Read the model definition and answer for the solid it produces. Units are mm, in the model's axes. Coordinates: 2 decimals unless noted, no trailing zeros.
Q1. The mould has two halves that part along X. Classify faces 1 (the face through (-47.083, -0.014, 44.087)), 2 (the face through (-70.4, 26.4, 2.6)), 3 (the face through (-85.32, 15.44, -56.24)): pulls with the +X half, pulls with the -X half, needs draft (parallel to the pull), parting line crosses it, or undercut.
Q2. Straight lines are drawn through the part: line 1 (Z direction, x = -100, y = 10); line 2 (Z direction, x = -55.5, y = 20.75); line 3 (Z direction, x = -84, y = 9.75). For each, find the intervals that lie inside material, in ascending order.
Q3. Flat-ended cylindrical pins translate along their axes: P1, Ø1.5, axis at x = -83, y = 21, coming from the +Z side; P2, Ø8.5, axis at x = -54.5, z = -26.5, coming from the +Y side; P3, Ø10, axis at x = -59.5, y = 7.5, coming from the +Z side. Find the tip coordinate at first contact, or state that the pin passes through.
Q4. Section A-A (y = 19) is taken. Count the separate pieces of the cut face and the enclosed holes in it, then the cut area to 3 significant figures.
from build123d import *

# Parameters (mm, degrees)
BOSS_EXTRUDE1_DEPTH = 1
BOSS_EXTRUDE2_DEPTH = 25.4
SKETCH4_R           = 14.351
CUT_EXTRUDE1_DEPTH  = 25.4
SKETCH4_4_R         = 19.177
CUT_EXTRUDE2_DEPTH  = 22.225
LPATTERN1_COUNT     = 3
LPATTERN1_PITCH     = 78
SPLIT3_START        = -1
SPLIT3_DEPTH        = 27.4


# Read off the part's stored shape, not the designer's step: Split3
with BuildPart() as part:
    # Sketch1 → Boss-Extrude1 (new, symmetric)
    with BuildSketch(Plane(origin=(0, 0, 0), x_dir=(1, 0, 0), z_dir=(0, 1, 0))):
        Polygon((118, 0), (-118, 0), (-118, -67.135), (118, -75), align=None)
        Polygon((-118, 67.135), (-118, 0), (118, 0), (118, 75), align=None)
    extrude(amount=BOSS_EXTRUDE1_DEPTH, both=True)

    # Sketch3 → Boss-Extrude2 (add)
    with BuildSketch(Plane(origin=(0, 1, 0), x_dir=(1, 0, 0), z_dir=(0, 1, 0))):
        Polygon((-84.001477372, 20.6375), (-73.002954744, 39.6875), (-84.001477372, 58.7375), (-105.998522628, 58.7375), (-116.997045256, 39.6875), (-105.998522628, 20.6375), align=None)
        Polygon((-38.632571531, 19.84375), (-49.631094159, 0.79375), (-71.628139415, 0.79375), (-82.626662043, 19.84375), (-71.628139415, 38.89375), (-49.631094159, 38.89375), align=None)
        Polygon((-84.001477372, -19.05), (-73.002954744, 0), (-84.001477372, 19.05), (-105.998522628, 19.05), (-116.997045256, 0), (-105.998522628, -19.05), align=None)
        Polygon((-105.998522628, -58.7375), (-84.001477372, -58.7375), (-73.002954744, -39.6875), (-84.001477372, -20.6375), (-105.998522628, -20.6375), (-116.997045256, -39.6875), align=None)
        Polygon((-71.628139415, -38.89375), (-49.631094159, -38.89375), (-38.632571531, -19.84375), (-49.631094159, -0.79375), (-71.628139415, -0.79375), (-82.626662043, -19.84375), align=None)
    boss_extrude2 = extrude(amount=BOSS_EXTRUDE2_DEPTH)

    # Sketch4 → Cut-Extrude1 (cut)
    with BuildSketch(Plane(origin=(0, 26.4, 0), x_dir=(1, 0, 0), z_dir=(0, 1, 0))):
        with Locations(Location((-95, 0, 0), (0, 0, 270))):
            Circle(SKETCH4_R)
        with Locations(Location((-95, -39.6875, 0), (0, 0, 270))):
            Circle(SKETCH4_R)
        with Locations(Location((-95, 39.6875, 0), (0, 0, 90))):
            Circle(SKETCH4_R)
        with Locations(Location((-60.629616787, 19.84375, 0), (0, 0, 270))):
            Circle(SKETCH4_R)
        with Locations(Location((-60.629616787, -19.84375, 0), (0, 0, 90))):
            Circle(SKETCH4_R)
    cut_extrude1 = extrude(amount=-CUT_EXTRUDE1_DEPTH, mode=Mode.SUBTRACT)

    # Sketch4<4> → Cut-Extrude2 (cut)
    with BuildSketch(Plane(origin=(0, 26.4, 0), x_dir=(1, 0, 0), z_dir=(0, 1, 0))):
        with Locations((-95, 0)):
            Circle(SKETCH4_4_R)
        with Locations((-95, -39.6875)):
            Circle(SKETCH4_4_R)
        with Locations((-95, 39.6875)):
            Circle(SKETCH4_4_R)
        with Locations((-60.629616787, 19.84375)):
            Circle(SKETCH4_4_R)
        with Locations((-60.629616787, -19.84375)):
            Circle(SKETCH4_4_R)
    cut_extrude2 = extrude(amount=-CUT_EXTRUDE2_DEPTH, mode=Mode.SUBTRACT)

    # LPattern1: Boss-Extrude2, Cut-Extrude1, Cut-Extrude2 ×3
    with Locations(*[(i * LPATTERN1_PITCH, 0, 0) for i in range(1, LPATTERN1_COUNT)]):
        add(boss_extrude2)
        add(cut_extrude1, mode=Mode.SUBTRACT)
        add(cut_extrude2, mode=Mode.SUBTRACT)

    # Split3 outline → Split3 (cut)
    with BuildSketch(Plane(origin=(0, 0, 0), x_dir=(1, 0, 0), z_dir=(0, 1, 0)).offset(SPLIT3_START)):
        Polygon((-44.543205596, 0), (-33.086411192, -19.84375), (-61.477571296, -69.018681787), (118, -75), (118, 75), (-61.477571296, 69.018681787), (-33.086411192, 19.84375), align=None)
    extrude(amount=SPLIT3_DEPTH, mode=Mode.SUBTRACT)


solid = part.part
Numbers:
1. face 1: pulls with the +X half
1. face 2: needs draft
1. face 3: undercut
2. line 1: z = -58.74 to -58.2, -21.17 to -20.64, -19.05 to -18.51, 18.51 to 19.05, 20.64 to 21.17, 58.2 to 58.74
2. line 2: z = -38.89 to -38.32, -1.37 to -0.79, 0.79 to 1.37, 38.32 to 38.89
2. line 3: z = -58.73 to -55.4, -23.98 to -20.64, -19.05 to -15.71, 15.71 to 19.05, 20.64 to 23.98, 55.4 to 58.73
3. P1: stops at z = 58.3
3. P2: stops at y = 1
3. P3: stops at z = 38.89
4. separate pieces: 30
4. enclosed holes: 0
4. area: 520 mm2
